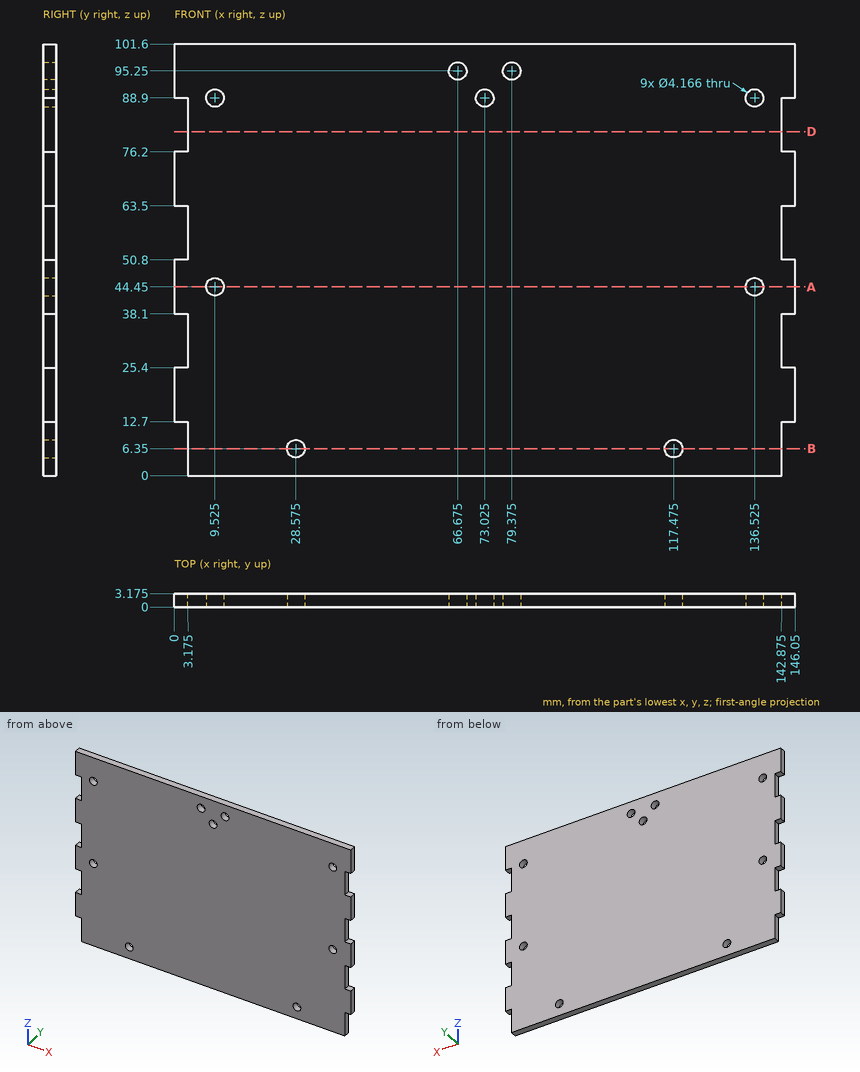
The figure shows three views and two pictorial views of one solid part (mm, origin at its lowest corner). Answer the questions. Give positions to 0.01 mm unless a question says otherwise; leave off trailing zeros. Loops run counter-clockwise (first coordinate to the right, second up) from the corner with the lowest first, then second, coordinate; pieces in that order, holes last. Notation, with made-up numbers: (17.25, -7) - (34.25, -7) arc R34 ccw to (34.25, 25) - close; hole circle Ø5 at (36.25, 40.25). An arc over 180 degrees is marked (long way). Answer in a Markdown table with one row per item.
(1) Section D-D (z = 81) is taken. Give the vertices of the cut face in (x, y) (1 decimal).
Results list:
| item | result |
|---|---|
| outline | (3.2, 0) - (142.9, 0) - (142.9, 3.2) - (3.2, 3.2) - close |
(2) Section A-A (z = 44.45) is taken. State how many separate pieces and enclosed holes the cut face has, and give its area (3 significant figures).
Results list:
| item | result |
|---|---|
| separate pieces | 3 |
| enclosed holes | 0 |
| area | 437 mm² |
(3) Consider L1, parallel to X at y = 1.5, z = 95.25; L2, parallel to X at y = 0.7, z = 44.45; L3, parallel to Z at x = 136, y = 0.4 (1 decimal). Determine where each line is inside the solid, lowest interval first. Write a range as [from, to].
Results list:
| item | result |
|---|---|
| L1 | x = [0, 64.59], [68.76, 77.29], [81.46, 146.05] |
| L2 | x = [0, 7.44], [11.61, 134.44], [138.61, 146.05] |
| L3 | z = [0, 42.4], [46.5, 86.9], [90.9, 101.6] |
(4) Flat-ended cylindrical pins translate along their axes: pin 1 Ø5 at (x, z) = (66.675, 95.25) entering from -Y; pin 2 Ø1.6 at (y, z) = (1.5, 5.5) entering from +X (3 decimals); pin 3 Ø1 at (x, y) = (2, 1.5) entering from -Z; pin 4 Ø3.5 at (x, z) = (28.575, 6.35) entering from -Y. Find the tip coordinate at first contact, or state that the pin passes through.
Results list:
| item | result |
|---|---|
| pin 1 | stops at y = 0 |
| pin 2 | stops at x = 142.875 |
| pin 3 | stops at z = 12.7 |
| pin 4 | passes through |
(5) Section B-B (z = 6.35) is taken. Give the vertices of the cut face in (x, y) (1 decimal), and give its area (3 significant figures).
Results list:
| item | result |
|---|---|
| outline | (3.2, 0) - (26.5, 0) - (26.5, 3.2) - (3.2, 3.2) - close; (30.7, 0) - (115.4, 0) - (115.4, 3.2) - (30.7, 3.2) - close; (119.6, 0) - (142.9, 0) - (142.9, 3.2) - (119.6, 3.2) - close |
| area | 417 mm² |
